Can you work these out from the drawing? Everything is in mm from the part's minimum corner. Round coordinates to 2 decimals unless told otherwise and drop trailing zeros. Order: outer loops, then holes, each group sorted by start corner. A loop starts at its lowest first (then second) coordinate and runs counter-clockwise, first axis right, second up. Notation, with made-up numbers: (-5.75, 70) - (14.25, 70) arc R32 ccw to (14.25, 100) - close; hole circle Ø5 at (32.25, 73.25). An arc over 180 degrees is marked (long way). Write item = value, one per line.
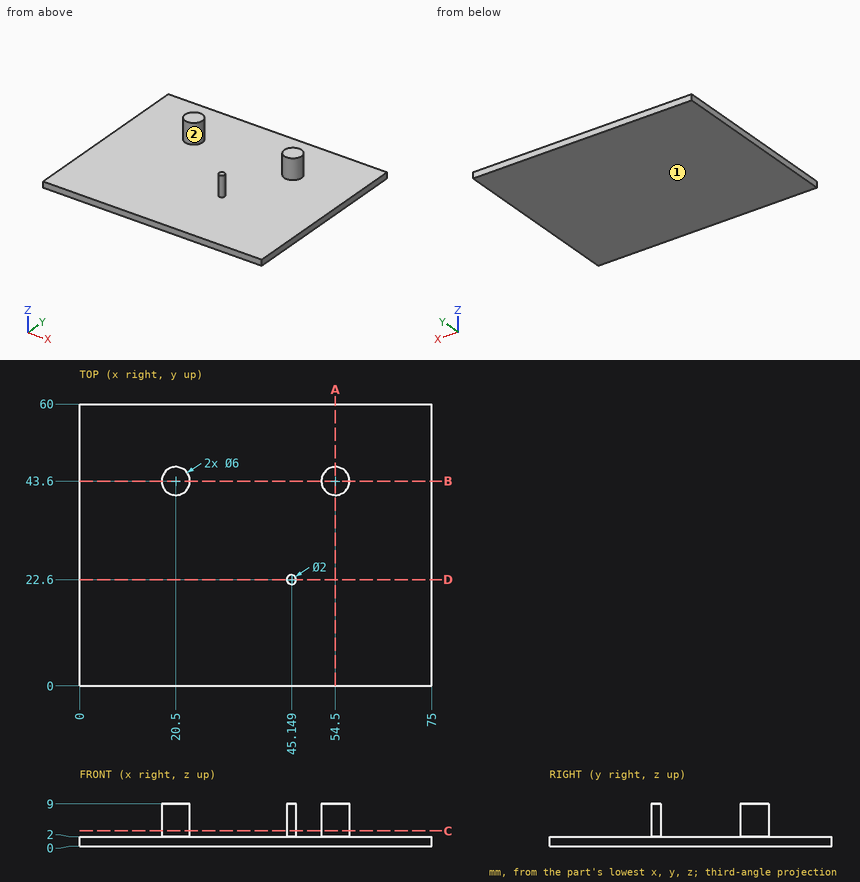
(1) If we section it at A-A (x = 54.5): Write out the boundary of the cut face in (y, z).
Computed:
outline = (0, 0) - (60, 0) - (60, 2) - (46.6, 2) - (46.6, 9) - (40.6, 9) - (40.6, 2) - (0, 2) - close
(2) Thinking about a two-plate mould opening in X: for the marked faces 1 and 2, which applies, +X half, -X half, draft (parallel to the pull), parting line (faces both ways), or undercut?
Computed:
face_1 = draft
face_2 = undercut
(3) If we section it at D-D (y = 22.6): Write out the boundary of the cut face in (x, z), plus the area to 3 significant figures.
Computed:
outline = (0, 0) - (75, 0) - (75, 2) - (46.15, 2) - (46.15, 9) - (44.15, 9) - (44.15, 2) - (0, 2) - close
area = 164 mm^2
(4) Will these pins go through, and if not, where does the flat tip stop? P1, Ø5, axis at y = 48, z = 6.5, coming from the +X side; P2, Ø8, axis at x = 32.5, y = 52, coming from the +Z side; P3, Ø1, axis at x = 21, z = 8, coming from the -Y side.
Computed:
P1 = 56.82
P2 = 2
P3 = 40.6
(5) If I drill on line 1 (Z direction, x = 10.5, y = 53); line 2 (X direction, y = 42, z = 5.5); line 3 (Y direction, x = 45, z = 2.5), over which ranges is the centre line in solid material (lowest first)? Write a range as from..to.
Computed:
line_1 = 0..2
line_2 = 17.96..23.04, 51.96..57.04
line_3 = 21.61..23.59
(6) If we section it at C-C (z = 3.25): Write out the boundary of the cut face in (x, y).
Computed:
outline = circle Ø6 at (20.5, 43.6); circle Ø2 at (45.15, 22.6); circle Ø6 at (54.5, 43.6)
(7) If we section it at B-B (y = 43.6): Write out the boundary of the cut face in (x, z), plus the area to 3 significant figures.
Computed:
outline = (0, 0) - (75, 0) - (75, 2) - (57.5, 2) - (57.5, 9) - (51.5, 9) - (51.5, 2) - (23.5, 2) - (23.5, 9) - (17.5, 9) - (17.5, 2) - (0, 2) - close
area = 234 mm^2
